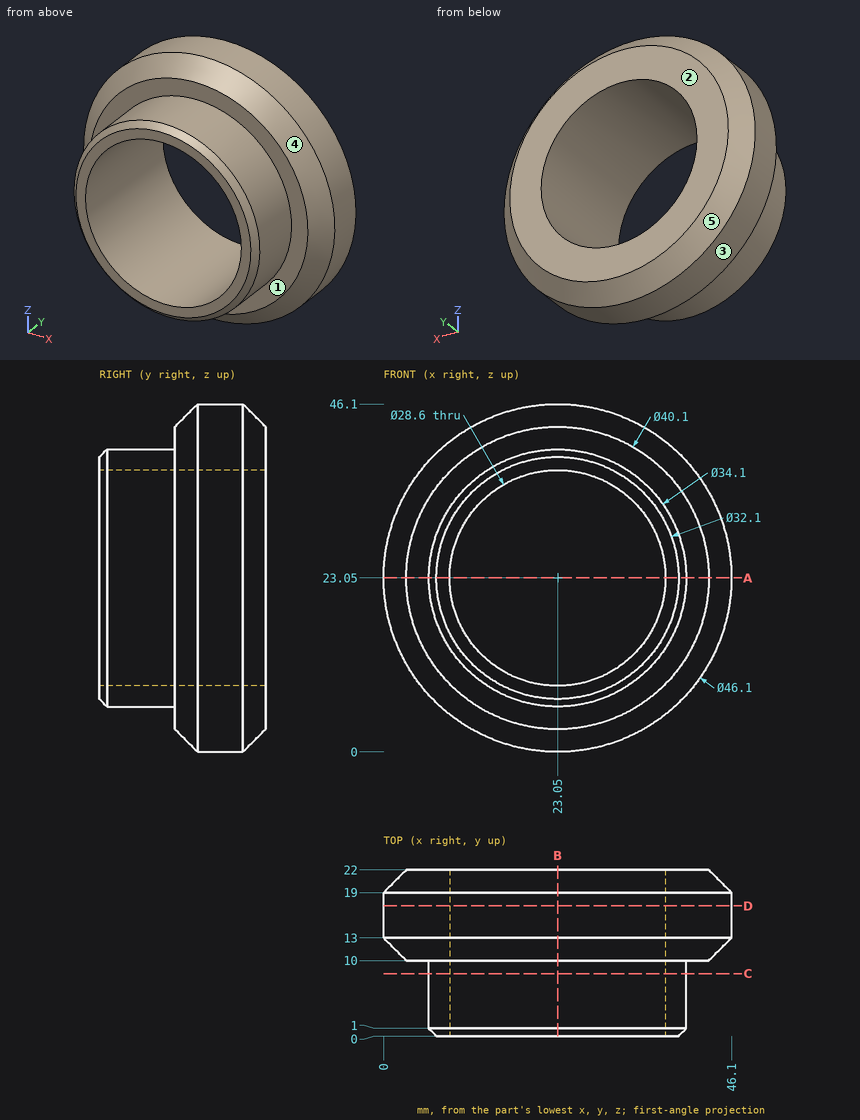
Verification items for this drawing (mm, ordinates from the low corner). A direction names the side the tool comes from. Coordinates: 2 decimals unless noted, no trailing zeros. Order: outer loops, then holes, each group sorted by start corner. A loop starts at its lowest first (then second) coordinate and runs counter-clockwise, first axis right, second up. Notation, with made-up numbers: (18, -4) - (30, -4) arc R22 cw to (30, 16) - close; hole circle Ø10 at (-37, -6.75). An arc over 180 degrees is marked (long way). Use one line per item in the form item = value.
1. Scan lines: line 1 (Z direction, x = 23.05, y = 8.75); line 2 (X direction, y = 2, z = 23.5); line 3 (X direction, y = 13, z = 23.05). Record each from-to range of solid material in increasing order.
Here are the results:
line_1 = 6 to 8.75, 37.35 to 40.1
line_2 = 6.01 to 8.76, 37.34 to 40.09
line_3 = 0 to 8.75, 37.35 to 46.1
2. Section check A-A (z = 23.05). Record the boundary of the cut face in (x, y).
Here are the results:
outline = (0, 13) - (3, 10) - (6, 10) - (6, 1) - (7, 0) - (8.75, 0) - (8.75, 22) - (3, 22) - (0, 19) - close; (37.35, 0) - (39.1, 0) - (40.1, 1) - (40.1, 10) - (43.1, 10) - (46.1, 13) - (46.1, 19) - (43.1, 22) - (37.35, 22) - close
3. Section check D-D (y = 17.25). Record the boundary of the cut face in (x, z).
Here are the results:
outline = circle Ø46.1 at (23.05, 23.05); hole circle Ø28.6 at (23.05, 23.05)
4. Section check C-C (y = 8.25). Record the boundary of the cut face in (x, z).
Here are the results:
outline = circle Ø34.1 at (23.05, 23.05); hole circle Ø28.6 at (23.05, 23.05)
5. Access from +Z, -Z, +X, -X, +Y, -Y to the whole of each face (thin tool, end or side, straight path). Record for the marked faces 1 and 2.
Here are the results:
face_1 = -Y
face_2 = +Z, -Z, +X, -X, +Y
6. Draft check along Y on the marked faces 3, 4 and 5. Enter one of: pulls with the +Y half, pulls with the -Y half, needs draft (parallel to the pull), parting line crosses it, or undercut.
Here are the results:
face_3 = needs draft
face_4 = pulls with the -Y half
face_5 = pulls with the +Y half
7. Section check B-B (x = 23.05). Record the boundary of the cut face in (y, z).
Here are the results:
outline = (0, 7) - (1, 6) - (10, 6) - (10, 3) - (13, 0) - (19, 0) - (22, 3) - (22, 8.75) - (0, 8.75) - close; (0, 37.35) - (22, 37.35) - (22, 43.1) - (19, 46.1) - (13, 46.1) - (10, 43.1) - (10, 40.1) - (1, 40.1) - (0, 39.1) - close
8. Gauge pin test, flat ends, axial feed: pin 1 (3 mm diameter, centred on x = 9, y = 16, fed in from +Z); pin 2 (1.5 mm diameter, centred on x = 27.5, y = 10, fed in from -Z); pin 3 (3 mm diameter, centred on y = 6, z = 19, fed in from +X). Record the tip position at first contact, or that the pin passes through.
Here are the results:
pin_1 = 42.38
pin_2 = 2.71
pin_3 = 39.91
